Read the model definition and answer for the solid it produces. Units are mm, in the model's axes. Coordinates: 2 decimals unless noted, no trailing zeros. Order: outer loops, then holes, each group sorted by start corner. A loop starts at its lowest first (then second) coordinate and runs counter-clockwise, first axis right, second up. Notation, with made-up numbers: M 68.5,57 L 109.5,57 A31 cw 109.5,87 Z; hole C -10.5,18.5 d6. An arc over 180 degrees is marked long. Put each result on its own line as item: value.
from build123d import *

# Parameters (mm, degrees)
F0_R     = 3.175
F1_DEPTH = 3.175
F2_R     = 1.524


with BuildPart() as f1:
    # F0 (on Top) → F1 (new body)
    with BuildSketch(Plane.XY):
        with BuildLine():
            Line((-71.123174, -70.829025), (49.116155, -70.829025))
            ThreePointArc((49.116155, -70.829025), (61.042759, -62.493211), (57.312992, -48.428414))
            Line((57.312992, -48.428414), (-62.926338, 53.171586))
            ThreePointArc((-62.926338, 53.171586), (-76.470612, 54.990303), (-83.823174, 43.470975))
            Line((-83.823174, 43.470975), (-83.823174, -58.129025))
            ThreePointArc((-83.823174, -58.129025), (-80.10343, -67.109281), (-71.123174, -70.829025))
        make_face()
        with Locations((-71.123174, -58.129025)):
            Circle(F0_R, mode=Mode.SUBTRACT)
        with Locations((49.116155, -58.129025)):
            Circle(F0_R, mode=Mode.SUBTRACT)
        with Locations((-71.123174, 43.470975)):
            Circle(F0_R, mode=Mode.SUBTRACT)
    extrude(amount=F1_DEPTH)

    # F2
    f2_edges = [f1.edges().sort_by_distance(p)[0] for p in [
        (-83.823174, -7.329025, 3.175),
    ]]
    fillet(f2_edges, radius=F2_R)


solid = f1.part
Q1. Consider line 1 along X through (y, z) = (-56.5, 0.7); line 2 along Y through (x, z) = (33.5, 0.55); line 3 along X through (y, z) = (18, 1.65). Determine where each line is inside the solid, lowest interval first.
Answers below:
line 1: x = -83.82 to -73.85, -68.4 to 46.39, 51.84 to 61.71
line 2: y = -70.83 to -28.31
line 3: x = -83.82 to -21.3
Q2. For a pull along Y with two mould halves and no side action, classify faces 1 (the face through (-71.54, -54.98, 1.57)), 2 (the face through (-28, -21, 0)), 3 (the face through (-3.93, 2.75, 2.72)) as +Y half, -Y half, draft (parallel to the pull), parting line (faces both ways), or undercut.
Answers below:
face 1: undercut
face 2: draft
face 3: +Y half
Q3. Given pin 1 (1.5 mm diameter, centred on x = 43, z = 2.5, fed in from -Y); pin 2 (5 mm diameter, centred on x = -7, y = 10, fed in from -Z), each flat-ended and moving along its own axis, determine where each tip first touches the part or whether it passes through.
Answers below:
pin 1: stops at y = -70.83
pin 2: passes through
Q4. Find section A-A on z = 2.2. Write down the section's boundary in (x, y) (3 decimals).
Answers below:
outline: M -83.721,-58.129 A12.598 ccw -71.123,-70.727 L 49.116,-70.727 A12.598 ccw 57.247,-48.507 L -62.992,53.093 A12.598 ccw -83.721,43.471 Z; hole C -71.123,-58.129 d6.35; hole C -71.123,43.471 d6.35; hole C 49.116,-58.129 d6.35
